Autodesk Inventor part; units mm, degrees
ref_plane "YZ Plane" through (0, 0, 0) normal (1, 0, 0) x (0, 1, 0)
ref_plane "XZ Plane" through (0, 0, 0) normal (0, 1, 0) x (-1, 0, 0)
ref_plane "XY Plane" through (0, 0, 0) normal (0, 0, 1) x (1, 0, 0)
sketch "Sketch1" plane through (0, 0, 0) normal (0, 0, 1) x (1, 0, 0)
  circle A0 centre (0, 0) radius 2
  circle A1 centre (0, 0) radius 1
  line L0 (0, 0) -> (20, 0)
  circle A2 centre (20, 0) radius 1.5
  circle A3 centre (20, 0) radius 0.6
  line L1 (0.05, 1.9994) -> (20.0375, 1.4995)
  line L2 (0.05, -1.9994) -> (20.0375, -1.4995)
  dimension "d0" = 4
  dimension "d1" = 2
  dimension "d2" = 20
  dimension "d3" = 3
  dimension "d4" = 1.2
extrude "Extrusion1" add sketch "Sketch1" along normal mid plane 4.6
sketch "Sketch2" plane through (0, 0, 0) normal (0, 0, 1) x (1, 0, 0)
  line L0 (0, 0) -> (2, 0)
  line L1 (2, 0) -> (2, 1.9506)
  line L2 (20.0375, 1.4995) -> (0.05, 1.9994)
  line L3 (2, 0) -> (2, -1.9506)
  line L4 (0.05, -1.9994) -> (20.0375, -1.4995)
  circle A0 centre (0, 0) radius 2.5
  circle A1 centre (20, 0) radius 0.6
  circle A2 centre (20, 0) radius 6
  point P0 (2, -1.5)
  point P1 (2, 1.5)
  point P2 (1.5495, 1.9619)
  point P3 (1.5495, -1.9619)
  dimension "d7" = 2
  dimension "d8" = 5
  dimension "d10" = 12
extrude "Extrusion2" cut sketch "Sketch2" along normal mid plane 2.6 contours L3 A0 L1 | L1 A0 L3 | A0 L2 L1 | L3 L4 A0 | A2
fillet "Fillet1" radius 0.1 4 edges at (2, 1.5, 0) (2, -1.5, 0) (2, 1.9506, 0) (2, -1.9506, 0)
fillet "Fillet2" radius 0.2 2 edges at (14.2298, 1.6448, 0) (14.2298, -1.6448, 0)
properties part number "New_ThinArm_second"
The model under review builds one solid part; all positions refer to its coordinate system, in mm. A direction names the side the tool comes from. Coordinates: 2 decimals unless noted, no trailing zeros. Write each loop counter-clockwise with the first axis right and the second up, starting at its lowest first coordinate (ties: lowest second). Pieces come first, ordered by that corner, then holes. Notation, with made-up numbers: (48, 75.5) - (57, 75.5) arc R10 ccw to (57, 83.5) - close; hole circle Ø3 at (-38.5, 89.5). An arc over 180 degrees is marked (long way). Answer as CSV lines item,"result".
(1) We need section D-D (y = -1.2). Give the boundary of the cut face in (x, z), plus the area to 3 significant figures.
Data:
outline,"(-1.6, -2.3) - (20.9, -2.3) - (20.9, -1.3) - (14.12, -1.3) - (14.12, 1.3) - (20.9, 1.3) - (20.9, 2.3) - (-1.6, 2.3) - (-1.6, 1.3) - (2.19, 1.3) - (2.19, -1.3) - (-1.6, -1.3) - close"
area,"76.0 mm2"
(2) We need section B-B (x = 16). Give the boundary of the cut face in (y, z), plus the area to 3 significant figures.
Data:
outline,"(-1.6, -2.3) - (1.6, -2.3) - (1.6, -1.3) - (-1.6, -1.3) - close; (-1.6, 1.3) - (1.6, 1.3) - (1.6, 2.3) - (-1.6, 2.3) - close"
area,"6.40 mm2"
(3) We need section A-A (y = 0). Give the boundary of the cut face in (x, z), plus the area to 3 significant figures.
Data:
outline,"(-2, -2.3) - (-1, -2.3) - (-1, -1.3) - (-2, -1.3) - close; (-2, 1.3) - (-1, 1.3) - (-1, 2.3) - (-2, 2.3) - close; (1, -2.3) - (19.4, -2.3) - (19.4, -1.3) - (14, -1.3) - (14, 1.3) - (19.4, 1.3) - (19.4, 2.3) - (1, 2.3) - (1, 1.3) - (2.5, 1.3) - (2.5, -1.3) - (1, -1.3) - close; (20.6, -2.3) - (21.5, -2.3) - (21.5, -1.3) - (20.6, -1.3) - close; (20.6, 1.3) - (21.5, 1.3) - (21.5, 2.3) - (20.6, 2.3) - close"
area,"70.5 mm2"
(4) Mouldability with a two-part tool opening along Y and no side actions: class faces 1 (the cylindrical face through (0, 1, -2)), 2 (the cylindrical face through (21.5, 0, -1.8)), 3 (the flat face through (10, 0, -2.3)) as pulls with the +Y half, pulls with the -Y half, needs draft (parallel to the pull), parting line crosses it, or undercut.
Data:
face 1,"undercut"
face 2,"parting line crosses it"
face 3,"needs draft"
(5) We need section C-C (z = 1.65). Give the boundary of the cut face in (x, y).
Data:
outline,"(0.05, -2) - (20.04, -1.5) arc R1.5 ccw to (20.04, 1.5) - (0.05, 2) arc R2 ccw (long way) to start; hole circle Ø2 at (0, 0); hole circle Ø1.2 at (20, 0)"
(6) For line 1 along X through (y, z) = (0, -2); line 2 along Z through (x, y) = (1.75, 1.6); line 3 along X through (y, z) = (0.3, -1.55), list the stretches that pass through material, from the lowest coordinate up. Write a range as [from, to].
Data:
line 1,"x = [-2, -1], [1, 19.4], [20.6, 21.5]"
line 2,"z = [-2.3, -1.3], [1.3, 2.3]"
line 3,"x = [-1.98, -0.95], [0.95, 19.48], [20.52, 21.47]"
(7) Tool access review of faces 4 (the cylindrical face through (2.5, 0, 0)), 5 (the cylindrical face through (20.554, 0.23, 1.793)), 6 (the cylindrical face through (14, 0, 0)): name each direction out of +Z, -Z, +X, -X, +Y, -Y from which nothing blocks a thin tool from reaching the whole face with its end or side.
Data:
face 4,"-X"
face 5,"+Z, -Z"
face 6,"+X"
